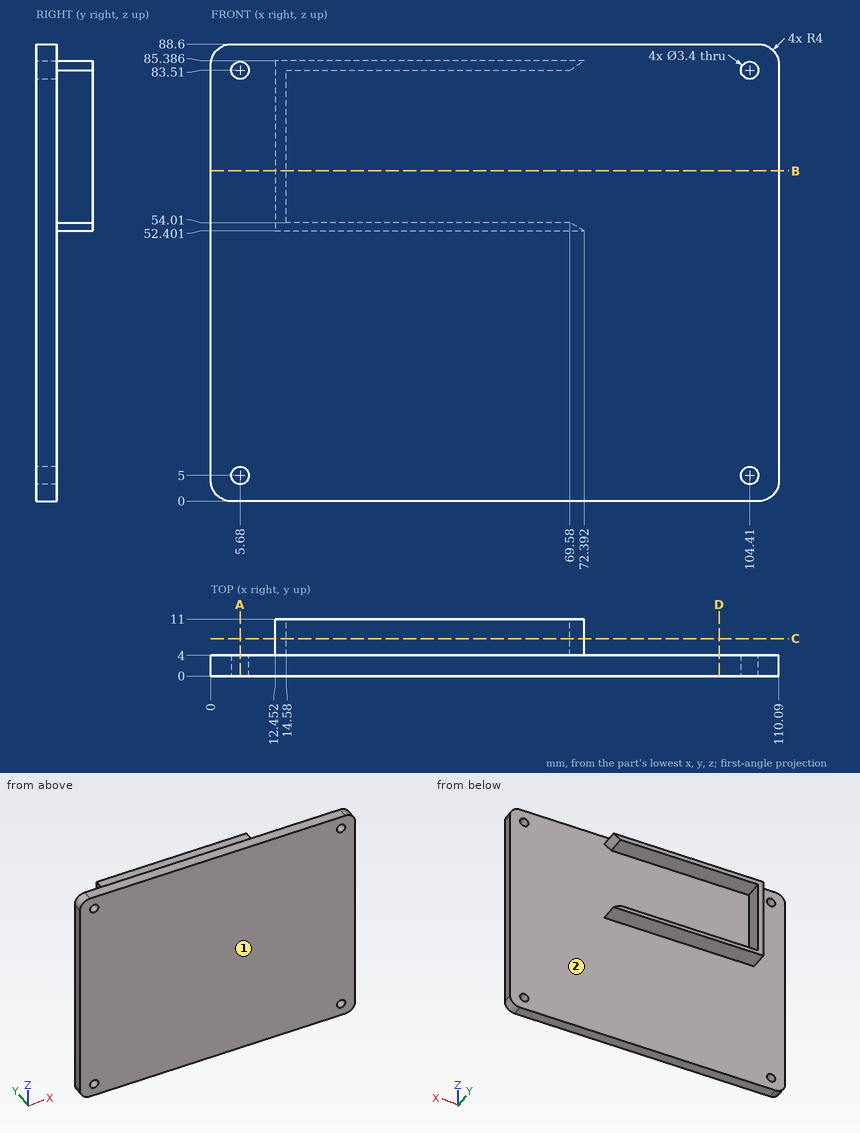
Answer from the drawing. Dimensions are ordinates in mm from the lowest x, y and z of the part. Coordinates: 2 decimals unless noted, no trailing zeros. Loops run counter-clockwise (first coordinate to the right, second up) from the corner with the lowest first, then second, coordinate; pieces in that order, holes last. Notation, with made-up numbers: (28, 31) - (72, 31) arc R25 ccw to (72, 50) - close; hole circle Ø5 at (0, 74). An arc over 180 degrees is marked (long way). Answer in a Markdown table with one row per item.
1. Straight lines are drawn through the part: line 1 (Z direction, x = 5.68, y = 1.05); line 2 (X direction, y = 3.1, z = 5); line 3 (X direction, y = 3.75, z = 85) (1 decimal). For each, find the intervals that lie inside material, in ascending order.
Conclusion:
| item | result |
|---|---|
| line 1 | z = 0 to 3.3, 6.7 to 81.81, 85.21 to 88.6 |
| line 2 | x = 0 to 3.98, 7.38 to 102.71, 106.11 to 110.09 |
| line 3 | x = 0 to 4.9, 6.5 to 103.6, 105.2 to 110.1 |
2. Find section A-A, the plane x = 5.68. Write down the section's boundary in (y, z), then the cut area to 3 significant figures.
Conclusion:
| item | result |
|---|---|
| outline | (0, 0) - (4, 0) - (4, 3.3) - (0, 3.3) - close; (0, 6.7) - (4, 6.7) - (4, 81.81) - (0, 81.81) - close; (0, 85.21) - (4, 85.21) - (4, 88.6) - (0, 88.6) - close |
| area | 327 mm² |
3. Find section B-B, the plane z = 64. Write down the section's boundary in (x, y), then the cut area to 3 significant figures.
Conclusion:
| item | result |
|---|---|
| outline | (0, 0) - (110.09, 0) - (110.09, 4) - (14.58, 4) - (14.58, 11) - (12.45, 11) - (12.45, 4) - (0, 4) - close |
| area | 455 mm² |
4. Find section C-C, the plane y = 7.25. Write down the section's boundary in (x, z) (1 decimal).
Conclusion:
| item | result |
|---|---|
| outline | (12.5, 52.4) - (72.4, 52.4) - (69.6, 54) - (14.6, 54) - (14.6, 83.5) - (69.6, 83.5) - (72.4, 85.4) - (12.5, 85.4) - close |
5. Given pin 1 (2 mm diameter, centred on x = 32, y = 7.5, fed in from -Z); pin 2 (5.5 mm diameter, centred on x = 104.41, z = 5, fed in from +Y); pin 3 (3 mm diameter, centred on x = 5.68, z = 5, fed in from -Y); pin 4 (6 mm diameter, centred on x = 20, y = 9.5, fed in from +Z), each flat-ended and moving along its own axis, determine where each tip first touches the part or whether it passes through.
Conclusion:
| item | result |
|---|---|
| pin 1 | stops at z = 52.4 |
| pin 2 | stops at y = 4 |
| pin 3 | passes through |
| pin 4 | stops at z = 85.39 |
6. Find section D-D, the plane x = 98.5. Write down the section's boundary in (y, z).
Conclusion:
| item | result |
|---|---|
| outline | (0, 0) - (4, 0) - (4, 88.6) - (0, 88.6) - close |
7. Determine the mould class of the marked faces 1 and 2 for opening direction Z: +Z half, -Z half, draft (parallel to the pull), parting line (faces both ways), or undercut.
Conclusion:
| item | result |
|---|---|
| face 1 | draft |
| face 2 | undercut |
